from build123d import *

# Parameters (mm, degrees)
SKETCH1_W           = 16
SKETCH1_H           = 16
BOSS_EXTRUDE1_DEPTH = 5
SHELL1_T            = -1
SKETCH2_R           = 2.7
SKETCH2_R_2         = 1.7
BOSS_EXTRUDE2_DEPTH = 4
SKETCH3_W           = 8
SKETCH3_H           = 5
BOSS_EXTRUDE3_DEPTH = 10
SKETCH4_W           = 8
SKETCH4_H           = 5
BOSS_EXTRUDE4_DEPTH = 10
SHELL2_START        = -17
SHELL2_OUTLINE_W    = 4
SHELL2_OUTLINE_H    = 6
SHELL2_DEPTH        = 9
SHELL2_START_2      = 8
SHELL2_2_OUTLINE_W  = 4
SHELL2_2_OUTLINE_H  = 6
SHELL2_2_DEPTH      = 9
BOSS_EXTRUDE5_DEPTH = 10


# Read off the part's stored shape, not the designer's step: Shell2
with BuildPart() as part:
    # Sketch1 → Boss-Extrude1 (new body)
    with BuildSketch(Plane(origin=(0, 0, 0), x_dir=(1, 0, 0), z_dir=(0, 1, 0))):
        Rectangle(SKETCH1_W, SKETCH1_H)
    extrude(amount=BOSS_EXTRUDE1_DEPTH)

    # Shell1
    shell1_openings = [part.faces().sort_by_distance(p)[0] for p in [
        (0, 0, 0),
    ]]
    offset(amount=SHELL1_T, openings=shell1_openings, kind=Kind.INTERSECTION)

    # Sketch2 → Boss-Extrude2 (add)
    with BuildSketch(Plane.XZ.offset(-4)):
        with Locations(Location((0, 0, 0), (0, 0, 90))):
            Circle(SKETCH2_R)
        with Locations(Location((0, 0, 0), (0, 0, 90))):
            Circle(SKETCH2_R_2, mode=Mode.SUBTRACT)
    extrude(amount=BOSS_EXTRUDE2_DEPTH)

    # Sketch3 → Boss-Extrude3 (add)
    with BuildSketch(Plane.ZY.offset(8)):
        with Locations((0, 2.5)):
            Rectangle(SKETCH3_W, SKETCH3_H)
    extrude(amount=BOSS_EXTRUDE3_DEPTH)

    # Sketch4 → Boss-Extrude4 (add)
    with BuildSketch(Plane(origin=(8, 0, 0), x_dir=(0, 0, -1), z_dir=(1, 0, 0))):
        with Locations((0, 2.5)):
            Rectangle(SKETCH4_W, SKETCH4_H)
    extrude(amount=BOSS_EXTRUDE4_DEPTH)

    # Shell2 outline → Shell2 (cut)
    with BuildSketch(Plane.YZ.offset(SHELL2_START)):
        with Locations((2, 0)):
            Rectangle(SHELL2_OUTLINE_W, SHELL2_OUTLINE_H)
    extrude(amount=SHELL2_DEPTH, mode=Mode.SUBTRACT)

    # Shell2 2 outline → Shell2 2 (cut)
    with BuildSketch(Plane.YZ.offset(SHELL2_START_2)):
        with Locations((2, 0)):
            Rectangle(SHELL2_2_OUTLINE_W, SHELL2_2_OUTLINE_H)
    extrude(amount=SHELL2_2_DEPTH, mode=Mode.SUBTRACT)

    # Sketch5 → Boss-Extrude5 (add)
    with BuildSketch(Plane(origin=(8, 0, 0), x_dir=(0, 0, -1), z_dir=(1, 0, 0))):
        with BuildLine():
            Line((4, 0), (8, 0))
            ThreePointArc((8, 0), (6.876952648, 3.201562119), (4, 5))
            Line((4, 5), (4, 0))
        make_face()
        with BuildLine():
            Line((-4, 0), (-8, 0))
            ThreePointArc((-8, 0), (-6.876952648, 3.201562119), (-4, 5))
            Line((-4, 5), (-4, 0))
        make_face()
    boss_extrude5 = extrude(amount=BOSS_EXTRUDE5_DEPTH)

    # Mirror2: Boss-Extrude5 across plane
    add(boss_extrude5.mirror(Plane(origin=(0, 0, 0), x_dir=(0, 0, 1), z_dir=(1, 0, 0))))


solid = part.part
Can you work these out from the model? Positions are in its coordinate system, mm. A direction names the side the tool comes from. Give positions to 0.01 mm unless a question says otherwise; leave off trailing zeros. Order: outer loops, then holes, each group sorted by start corner. A loop starts at its lowest first (then second) coordinate and runs counter-clockwise, first axis right, second up. Notation, with made-up numbers: M -32,-7 L -14,-7 A15 ccw -14,2 Z; hole C -33.75,22 d1. An arc over 180 degrees is marked long. Use one line per item in the form item = value. Start each with the question number.
Item 1: We'd pull the mould along X, two halves only. Please class faces 1 (the flat face through (8, 4, -7)), 2 (the flat face through (0, 2, -7)), 3 (the flat face through (0, 2, -8)): +X half, -X half, draft (parallel to the pull), parting line (faces both ways), or undercut.
Item 2: If we section it at A-A (y = 2.55): Write out the boundary of the cut face in (x, z).
Item 3: For faces 4 (the flat face through (-8, 4, -7)), 5 (the flat face through (-8, 4, 7)), 6 (the flat face through (0, 2, 8)), 7 (the cylindrical face through (12.93, 3.16, 6.91)), 8 (the flat face through (12, 4, 0)), which set-ups out of +Z, -Z, +X, -X, +Y, -Y let a thin tool reach every point of the face, with its end or its side?
Item 4: If we section it at C-C (y = 0.5): State how many separate pieces and enclosed holes the cut face has, then the cut area to 3 significant figures.
Item 5: If I drill on line 1 along X through (y, z) = (3.6, -2.75); line 2 along X through (y, z) = (2.5, 0); line 3 along X through (y, z) = (1.25, -4), over which ranges is the centre line in solid material (lowest first)?
Item 6: Will these pins go through, and if not, where does the flat tip stop? pin 1 Ø1.2 at (x, y) = (-13.5, 2.5) entering from +Z; pin 2 Ø1.7 at (x, z) = (0.5, -0.5) entering from -Y; pin 3 Ø1.2 at (x, y) = (-13, 1.5) entering from -Z.
Item 7: If we section it at D-D (z = 0): Write out the boundary of the cut face in (x, y), then the cut area to 3 significant figures.
Item 8: If we section it at B-B (x = 0): Write out the boundary of the cut face in (y, z), then the cut area to 3 significant figures.
Outcome:
q1.face_1 = +X half
q1.face_2 = undercut
q1.face_3 = draft
q2.outline = M -18,-7.32 L -8,-7.32 L -8,-8 L 8,-8 L 8,-7.32 L 18,-7.32 L 18,7.32 L 8,7.32 L 8,8 L -8,8 L -8,7.32 L -18,7.32 Z; C 0,0 d5.4; hole M -17,-3 L -8,-3 L -8,3 L -17,3 Z; hole M -7,-7 L 7,-7 L 7,7 L -7,7 Z; hole C 0,0 d3.4; hole M 8,-3 L 17,-3 L 17,3 L 8,3 Z
q3.face_4 = -Z, -X, +Y
q3.face_5 = +Z, -X, +Y
q3.face_6 = +Z, +X, -X, +Y, -Y
q3.face_7 = +Z, +X, +Y
q3.face_8 = -Y
q4.separate_pieces = 2
q4.enclosed_holes = 4
q4.area = 285 mm2
q5.line_1 = -18 to -17, -8 to -7, 7 to 8, 17 to 18
q5.line_2 = -18 to -17, -8 to -7, -2.7 to -1.7, 1.7 to 2.7, 7 to 8, 17 to 18
q5.line_3 = -18 to -7, 7 to 18
q6.pin_1 = 7.63
q6.pin_2 = 4
q6.pin_3 = -7.92
q7.outline = M -18,0 L -17,0 L -17,4 L -8,4 L -8,0 L -7,0 L -7,4 L -2.7,4 L -2.7,0 L -1.7,0 L -1.7,4 L 1.7,4 L 1.7,0 L 2.7,0 L 2.7,4 L 7,4 L 7,0 L 8,0 L 8,4 L 17,4 L 17,0 L 18,0 L 18,5 L -18,5 Z
q7.area = 60.0 mm2
q8.outline = M 0,-8 L 5,-8 L 5,8 L 0,8 L 0,7 L 4,7 L 4,2.7 L 0,2.7 L 0,1.7 L 4,1.7 L 4,-1.7 L 0,-1.7 L 0,-2.7 L 4,-2.7 L 4,-7 L 0,-7 Z
q8.area = 32.0 mm2
